```python
from build123d import *

# Parameters (mm, degrees)
IZIM1_R                     = 1.5
IZIM1_R_2                   = 0.75
Y_KSEKLIK_EKSTR_ZYON1_DEPTH = 2
IZIM2_R                     = 4.5
IZIM2_R_2                   = 2.75
Y_KSEKLIK_EKSTR_ZYON2_DEPTH = 4


with BuildPart() as part:
    # Çizim1 → Yükseklik-Ekstrüzyon1 (new body)
    with BuildSketch(Plane.XY):
        with BuildLine():
            Line((-16.933536585, 2.442404289), (-1.280487805, 5.861770294))
            ThreePointArc((-1.280487805, 5.861770294), (0, 6), (1.280487805, 5.861770294))
            Line((1.280487805, 5.861770294), (16.933536585, 2.442404289))
            ThreePointArc((16.933536585, 2.442404289), (18.9, 0), (16.933536585, -2.442404289))
            Line((16.933536585, -2.442404289), (1.280487805, -5.861770294))
            ThreePointArc((1.280487805, -5.861770294), (0, -6), (-1.280487805, -5.861770294))
            Line((-1.280487805, -5.861770294), (-16.933536585, -2.442404289))
            ThreePointArc((-16.933536585, -2.442404289), (-18.9, 0), (-16.933536585, 2.442404289))
        make_face()
        Circle(IZIM1_R, mode=Mode.SUBTRACT)
        with Locations((7.4, 0)):
            Circle(IZIM1_R_2, mode=Mode.SUBTRACT)
        with Locations((10.4, 0)):
            Circle(IZIM1_R_2, mode=Mode.SUBTRACT)
        with Locations((13.4, 0)):
            Circle(IZIM1_R_2, mode=Mode.SUBTRACT)
        with Locations((16.4, 0)):
            Circle(IZIM1_R_2, mode=Mode.SUBTRACT)
        with Locations((-7.4, 0)):
            Circle(IZIM1_R_2, mode=Mode.SUBTRACT)
        with Locations((-10.4, 0)):
            Circle(IZIM1_R_2, mode=Mode.SUBTRACT)
        with Locations((-13.4, 0)):
            Circle(IZIM1_R_2, mode=Mode.SUBTRACT)
        with Locations((-16.4, 0)):
            Circle(IZIM1_R_2, mode=Mode.SUBTRACT)
    extrude(amount=Y_KSEKLIK_EKSTR_ZYON1_DEPTH)

    # Çizim2 → Yükseklik-Ekstrüzyon2 (add)
    with BuildSketch(Plane.XY.offset(2)):
        Circle(IZIM2_R)
        Circle(IZIM2_R_2, mode=Mode.SUBTRACT)
    extrude(amount=Y_KSEKLIK_EKSTR_ZYON2_DEPTH)


solid = part.part
```
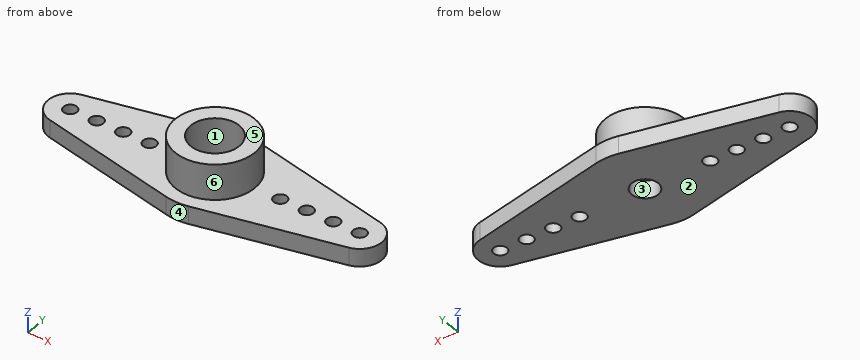
Design review of the part built by this model. Coordinates are the model's own, in mm. Face numbers are marked on the shaded views. A direction names the side the tool comes from. Coordinates: 2 decimals unless noted, no trailing zeros. Order: outer loops, then holes, each group sorted by start corner. A loop starts at its lowest first (then second) coordinate and runs counter-clockwise, first axis right, second up. Notation, with made-up numbers: (41.25, 15.25) - (66.25, 15.25) arc R23 cw to (66.25, 50.25) - close; hole circle Ø3 at (75.25, 75). An arc over 180 degrees is marked (long way). Answer in a Markdown table with one row per item.
(1) For the marked faces 5 and 6, list the 3-axis set-ups (+Z, -Z, +X, -X, +Y, -Y) from which the entire face can be reached by the end or side of a thin tool; tool diameter is ignored.
Checked values:
| item | result |
|---|---|
| face 5 | +Z, +X, -X, +Y, -Y |
| face 6 | +Z |
(2) Consider section B-B on z = 1.2. Give the number of separate pieces and of enclosed holes in the cut face, plus the area to 3 significant figures.
Checked values:
| item | result |
|---|---|
| separate pieces | 1 |
| enclosed holes | 9 |
| area | 284 mm^2 |
(3) Wall thickness on line 1 along Y through (x, z) = (0, 1.5); line 2 along Z through (x, y) = (6, -3); line 3 along Y through (x, z) = (10.4, 1.2): over which ranges is each line inside the solid? List them lowest first. Write a range as from..to.
Checked values:
| item | result |
|---|---|
| line 1 | -6..-1.5, 1.5..6 |
| line 2 | 0..2 |
| line 3 | -3.87..-0.75, 0.75..3.87 |
(4) The part is to be moulded in two halves that separate along X. For the marked faces 1, 2, 3 and 4, say which applies: released by +X, released by -X, zero draft, split by the parting line, or undercut.
Checked values:
| item | result |
|---|---|
| face 1 | undercut |
| face 2 | zero draft |
| face 3 | undercut |
| face 4 | split by the parting line |
(5) Clearance check with flat-ended pins moving along their axes: pin 1 (3 mm diameter, centred on y = -1, z = 4.5, fed in from +X); pin 2 (2 mm diameter, centred on x = -16.4, y = 0, fed in from +Z); pin 3 (1.5 mm diameter, centred on y = -1, z = 3, fed in from -X). State where each tip first meets the part, or that it passes through.
Checked values:
| item | result |
|---|---|
| pin 1 | x = 4.5 |
| pin 2 | z = 2 |
| pin 3 | x = -4.49 |
(6) Consider section A-A on x = 0. State the section outline as (y, z) points, plus the area to 3 significant figures.
Checked values:
| item | result |
|---|---|
| outline | (-6, 0) - (-1.5, 0) - (-1.5, 2) - (-2.75, 2) - (-2.75, 6) - (-4.5, 6) - (-4.5, 2) - (-6, 2) - close; (1.5, 0) - (6, 0) - (6, 2) - (4.5, 2) - (4.5, 6) - (2.75, 6) - (2.75, 2) - (1.5, 2) - close |
| area | 32.0 mm^2 |
(7) Consider section D-D on x = 10.5. State the section outline as (y, z) points.
Checked values:
| item | result |
|---|---|
| outline | (-3.85, 0) - (-0.74, 0) - (-0.74, 2) - (-3.85, 2) - close; (0.74, 0) - (3.85, 0) - (3.85, 2) - (0.74, 2) - close |
